from build123d import *

# Parameters (mm, degrees)
SKETCH1_R      = 17.5
EXTRUDE1_DEPTH = 14.2
FILLET1_R      = 0.75
SKETCH2_R      = 2.413
EXTRUDE2_DEPTH = 0.8
SKETCH3_R      = 5
EXTRUDE3_DEPTH = 2
SKETCH4_R      = 5
EXTRUDE4_DEPTH = 0.7
SKETCH5_R      = 1
EXTRUDE5_DEPTH = 11.5


with BuildPart() as part:
    # Sketch1 → Extrude1 (new body)
    with BuildSketch(Plane(origin=(0, 0, 0), x_dir=(1, 0, 0), z_dir=(0, 1, 0))):
        with Locations(Location((0, 0, 0), (0, 0, 270))):  # turned: the seam where the file's is
            Circle(SKETCH1_R)
    extrude(amount=EXTRUDE1_DEPTH)

    # Fillet1
    fillet1_edges = [part.edges().sort_by_distance(p)[0] for p in [
        (0, 0, -17.5),
        (0, 14.2, -17.5),
    ]]
    fillet(fillet1_edges, radius=FILLET1_R)

    # Sketch2 → Extrude2 (add)
    with BuildSketch(Plane(origin=(0, 14.2, 0), x_dir=(-1, 0, 0), z_dir=(0, 1, 0))):
        with BuildLine():
            Line((23.380952381, -3.21419753), (9.821428571, -13.25856481))
            ThreePointArc((9.821428571, -13.25856481), (0, -16.5), (-9.821428571, -13.25856481))
            Line((-9.821428571, -13.25856481), (-23.380952381, -3.21419753))
            ThreePointArc((-23.380952381, -3.21419753), (-25, 0), (-23.380952381, 3.21419753))
            Line((-23.380952381, 3.21419753), (-9.821428571, 13.25856481))
            ThreePointArc((-9.821428571, 13.25856481), (0, 16.5), (9.821428571, 13.25856481))
            Line((9.821428571, 13.25856481), (23.380952381, 3.21419753))
            ThreePointArc((23.380952381, 3.21419753), (25, 0), (23.380952381, -3.21419753))
        make_face()
        with Locations(Location((21, 0, 0), (0, 0, 90))):  # turned: the seam where the file's is
            Circle(SKETCH2_R, mode=Mode.SUBTRACT)
        with Locations(Location((-21, 0, 0), (0, 0, 270))):  # turned: the seam where the file's is
            Circle(SKETCH2_R, mode=Mode.SUBTRACT)
    extrude(amount=EXTRUDE2_DEPTH)

    # Sketch3 → Extrude3 (add)
    with BuildSketch(Plane.XZ):
        with Locations(Location((0, 0, 0), (0, 0, 90))):  # turned: the seam where the file's is
            Circle(SKETCH3_R)
    extrude(amount=EXTRUDE3_DEPTH)

    # Sketch4 → Extrude4 (add)
    with BuildSketch(Plane(origin=(0, 15, 0), x_dir=(-1, 0, 0), z_dir=(0, 1, 0))):
        with Locations(Location((0, 0, 0), (0, 0, 90))):  # turned: the seam where the file's is
            Circle(SKETCH4_R)
    extrude(amount=EXTRUDE4_DEPTH)

    # Sketch5 → Extrude5 (add)
    with BuildSketch(Plane(origin=(0, 15.7, 0), x_dir=(-1, 0, 0), z_dir=(0, 1, 0))):
        with Locations(Location((0, 0, 0), (0, 0, 90))):  # turned: the seam where the file's is
            Circle(SKETCH5_R)
    extrude(amount=EXTRUDE5_DEPTH)


solid = part.part
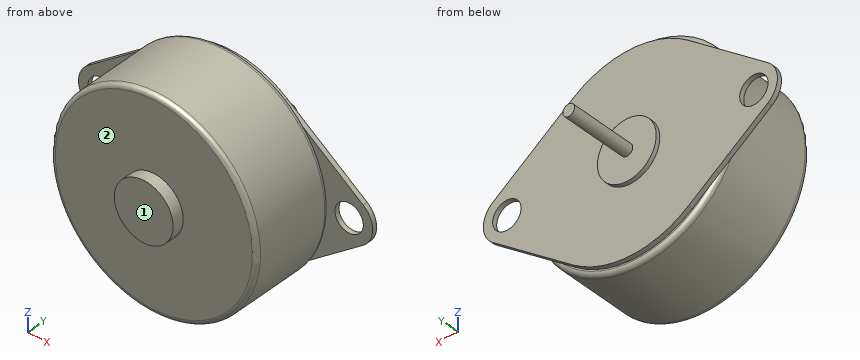
Part model, mm, in its own coordinate system. Face numbers are marked on the shaded views. A direction names the side the tool comes from. Give positions to 0.01 mm unless a question says otherwise; leave off trailing zeros. Order: outer loops, then holes, each group sorted by start corner. A loop starts at its lowest first (then second) coordinate and runs counter-clockwise, first axis right, second up. Notation, with made-up numbers: (60.25, 23.25) - (85.25, 23.25) arc R32 ccw to (85.25, 61.25) - close; hole circle Ø10 at (33, 1.25). An arc over 180 degrees is marked (long way). Use a Markdown table: item, result.
1) Probe L1, parallel to X at y = 14.85, z = 0; L2, parallel to Y at x = 1, z = -12.5; L3, parallel to Y at x = -16, z = -6.5. List the from-to ranges inside material, lowest first. Write a range as from..to.
Checked values:
| item | result |
|---|---|
| L1 | -25..-23.41, -18.59..18.59, 23.41..25 |
| L2 | 0..15 |
| L3 | 0.21..13.99, 14.2..15 |
2) Saw through at C-C on x = 0. List the corners of the cut face in (y, z), plus the area to 3 significant figures.
Checked values:
| item | result |
|---|---|
| outline | (-2, -5) - (0, -5) - (0, -16.75) arc R0.75 ccw to (0.75, -17.5) - (13.45, -17.5) arc R0.75 ccw to (14.2, -16.75) - (14.2, -16.5) - (15, -16.5) - (15, -5) - (15.7, -5) - (15.7, -1) - (27.2, -1) - (27.2, 1) - (15.7, 1) - (15.7, 5) - (15, 5) - (15, 16.5) - (14.2, 16.5) - (14.2, 16.75) arc R0.75 ccw to (13.45, 17.5) - (0.75, 17.5) arc R0.75 ccw to (0, 16.75) - (0, 5) - (-2, 5) - close |
| area | 573 mm² |
3) Saw through at D-D on y = 25.5. List the corners of the cut face in (x, z).
Checked values:
| item | result |
|---|---|
| outline | circle Ø2 at (0, 0) |
4) Flat gauge pins, fed straight in: P1, Ø1.6, axis at x = 1.5, z = -14, coming from the +Y side; P2, Ø4, axis at x = 18, z = 4.5, coming from the -Y side; P3, Ø8, axis at x = 11.5, y = 12.5, coming from the +Z side. Where does each tip first touch, or does it go through?
Checked values:
| item | result |
|---|---|
| P1 | y = 15 |
| P2 | y = 0 |
| P3 | z = 15.81 |
5) 3-axis set-ups, long thin cutter, end or side, ignore diameter. For the marked faces 1 and 2: which of +Z, -Z, +X, -X, +Y, -Y reach the whole face in a straight line?
Checked values:
| item | result |
|---|---|
| face 1 | +Z, -Z, +X, -X, -Y |
| face 2 | -Y |
6) Saw through at B-B on x = -20. List the corners of the cut face in (y, z), plus the area to 3 significant figures.
Checked values:
| item | result |
|---|---|
| outline | (14.2, -5.72) - (15, -5.72) - (15, -2.2) - (14.2, -2.2) - close; (14.2, 2.2) - (15, 2.2) - (15, 5.72) - (14.2, 5.72) - close |
| area | 5.64 mm² |
7) Saw through at A-A on z = 0. Count the separate pieces of the cut face and the enclosed holes in it, plus the area to 3 significant figures.
Checked values:
| item | result |
|---|---|
| separate pieces | 3 |
| enclosed holes | 0 |
| area | 579 mm² |
